Could you check a few things on this model? Use its own coordinates, in mm. A direction names the side the tool comes from. Round coordinates to 2 decimals unless told otherwise and drop trailing zeros. Order: outer loops, then holes, each group sorted by start corner. A loop starts at its lowest first (then second) coordinate and runs counter-clockwise, first axis right, second up. Notation, with made-up numbers: (-34.5, 81.25) - (-6.5, 81.25) arc R23 ccw to (-6.5, 100.25) - close; hole circle Ø10 at (-6.5, 35.5). An arc over 180 degrees is marked (long way). Return JSON: item names as keys, results as strings. Group by question number.
from build123d import *

# Parameters (mm, degrees)
SKETCH1_W                 = 100
SKETCH1_H                 = 126.094412
BOSS_EXTRUDE1_DEPTH       = 5
SLOTS_DEPTH               = 11
CUT_EXTRUDE5_DEPTH        = 3
CHAMFER2_SIZE             = 0.2
M5X0_8_TAPPED_HOLE2_D     = 4.2
SKETCH10_R                = 4.15
CUT_EXTRUDE4_DEPTH        = 5
M5X0_8_TAPPED_HOLE1_D     = 4.2
M5X0_8_TAPPED_HOLE1_DEPTH = 20
M5X0_8_TAPPED_HOLE1_TIP   = 1.2618073
CUT_EXTRUDE2_DEPTH        = 11
CUT_EXTRUDE3_DEPTH        = 11
FILLET1_R                 = 4
CHAMFER1_SIZE             = 2


with BuildPart() as part:
    # Sketch1 → Boss-Extrude1 (new body, symmetric)
    with BuildSketch(Plane(origin=(0, 0, 0), x_dir=(1, 0, 0), z_dir=(0, 1, 0))):
        with Locations((10, -5.047206)):
            Rectangle(SKETCH1_W, SKETCH1_H)
    extrude(amount=BOSS_EXTRUDE1_DEPTH, both=True)

    # Sketch3 → Slots (cut, through all)
    with BuildSketch(Plane(origin=(0, 5, 0), x_dir=(1, 0, 0), z_dir=(0, 1, 0))):
        with BuildLine():
            Line((-8.05, 0), (-8.05, -34.641016151))
            ThreePointArc((-8.05, -34.641016151), (0, -42.691016151), (8.05, -34.641016151))
            Line((8.05, -34.641016151), (8.05, 0))
            ThreePointArc((8.05, 0), (0, 8.05), (-8.05, 0))
        make_face()
        with BuildLine():
            Line((-11.95, 0), (-11.95, 20))
            ThreePointArc((-11.95, 20), (-8.449926035, 28.449926035), (0, 31.95))
            ThreePointArc((0, 31.95), (15.975, 27.669511651), (27.669511651, 15.975))
            ThreePointArc((27.669511651, 15.975), (38.666016151, 13.0284955), (41.612520652, 24.025))
            ThreePointArc((41.612520652, 24.025), (24.025, 41.612520652), (0, 48.05))
            ThreePointArc((0, 48.05), (-19.834345212, 39.834345212), (-28.05, 20))
            Line((-28.05, 20), (-28.05, 0))
            ThreePointArc((-28.05, 0), (-20, -8.05), (-11.95, 0))
        make_face()
    extrude(amount=-SLOTS_DEPTH, mode=Mode.SUBTRACT)

    # Sketch11 → Cut-Extrude5 (cut)
    with BuildSketch(Plane(origin=(0, 5, 0), x_dir=(1, 0, 0), z_dir=(0, 1, 0))):
        with BuildLine():
            Line((-10.15, 0), (-10.15, -34.641016151))
            ThreePointArc((-10.15, -34.641016151), (0, -44.791016151), (10.15, -34.641016151))
            Line((10.15, -34.641016151), (10.15, 0))
            ThreePointArc((10.15, 0), (0, 10.15), (-10.15, 0))
        make_face()
    extrude(amount=-CUT_EXTRUDE5_DEPTH, mode=Mode.SUBTRACT)

    # Chamfer2
    chamfer2_edges = [part.edges().sort_by_distance(p)[0] for p in [
        (0, 5, -10.15),
        (-10.15, 5, 17.320508076),
        (0, 5, 44.791016151),
        (10.15, 5, 17.320508076),
    ]]
    chamfer(chamfer2_edges, length=CHAMFER2_SIZE)

    # M5x0.8 Tapped Hole2 (through all)
    with Locations(Plane(origin=(0, 5, 0), x_dir=(1, 0, 0), z_dir=(0, 1, 0))):
        with Locations((-20, -34.641016151)):
            Hole(M5X0_8_TAPPED_HOLE2_D / 2)

    # Sketch10 → Cut-Extrude4 (cut)
    with BuildSketch(Plane(origin=(0, 5, 0), x_dir=(1, 0, 0), z_dir=(0, 1, 0))):
        with Locations((-20, -34.641016151)):
            Circle(SKETCH10_R)
    extrude(amount=-CUT_EXTRUDE4_DEPTH, mode=Mode.SUBTRACT)

    # M5x0.8 Tapped Hole1
    with Locations(Plane.XY.offset(68.094412)):
        with Locations((-15, 0), (35, 0)):
            Hole(M5X0_8_TAPPED_HOLE1_D / 2, depth=M5X0_8_TAPPED_HOLE1_DEPTH)
            with Locations((0, 0, -(M5X0_8_TAPPED_HOLE1_DEPTH + M5X0_8_TAPPED_HOLE1_TIP / 2))):  # 118° drill point
                Cone(0, M5X0_8_TAPPED_HOLE1_D / 2, M5X0_8_TAPPED_HOLE1_TIP, mode=Mode.SUBTRACT)

    # Sketch4 → Cut-Extrude2 (cut, through all)
    with BuildSketch(Plane(origin=(0, 5, 0), x_dir=(1, 0, 0), z_dir=(0, 1, 0))):
        Polygon((-40, 43), (-40, 58), (-25, 58), align=None)
    extrude(amount=-CUT_EXTRUDE2_DEPTH, mode=Mode.SUBTRACT)

    # Sketch5 → Cut-Extrude3 (cut, through all)
    with BuildSketch(Plane(origin=(0, 5, 0), x_dir=(1, 0, 0), z_dir=(0, 1, 0))):
        Polygon((25, 58), (60, 58), (60, 23), align=None)
    extrude(amount=-CUT_EXTRUDE3_DEPTH, mode=Mode.SUBTRACT)

    # Fillet1
    fillet1_edges = [part.edges().sort_by_distance(p)[0] for p in [
        (-25, 0, -58),
        (-40, 0, -43),
        (60, 0, -23),
        (25, 0, -58),
    ]]
    fillet(fillet1_edges, radius=FILLET1_R)

    # Chamfer1
    chamfer1_edges = [part.edges().sort_by_distance(p)[0] for p in [
        (60, 5, 23.375633125),
        (42.5, 5, -40.5),
        (0, 5, -58),
        (-32.5, 5, -50.5),
        (-40, 5, 13.375633125),
        (-39.69551813, 5, -42.87387948),
        (-24.87387948, 5, -57.69551813),
        (24.87387948, 5, -57.69551813),
        (59.69551813, 5, -22.87387948),
        (42.5, -5, -40.5),
        (-40, -5, 13.375633125),
        (-32.5, -5, -50.5),
        (0, -5, -58),
        (-39.69551813, -5, -42.87387948),
        (-24.87387948, -5, -57.69551813),
        (24.87387948, -5, -57.69551813),
        (59.69551813, -5, -22.87387948),
        (60, -5, 23.375633125),
    ]]
    chamfer(chamfer1_edges, length=CHAMFER1_SIZE)


solid = part.part
1) If I drill on line 1 along X through (y, z) = (0, 60.75); line 2 along Y through (x, z) = (35, 52.5); line 3 along Z through (x, y) = (-20, -3.05), over which ranges is the centre line in solid material (lowest first)? Write a range as from..to.
2) I want a section at B-B, the plane z = 5.5. List the corners of the cut face in (x, y) for me, plus the area to 3 significant figures.
3) I want a section at D-D, the plane x = 48. List the corners of the cut face in (y, z) for me, plus the area to 3 significant figures.
4) I want a section at C-C, the plane x = -20. List the corners of the cut face in (y, z) for me, plus the area to 3 significant figures.
5) Will these pins go through, and if not, where does the flat tip stop? pin 1 (0.8 mm diameter, centred on y = 4, z = 14, fed in from -X); pin 2 (7.5 mm diameter, centred on x = -20, z = 34.64, fed in from +Y); pin 3 (16 mm diameter, centred on x = -1.5, z = 5.5, fed in from +Y); pin 4 (6.5 mm diameter, centred on x = -18, z = 34.5, fed in from +Y).
6) For faces 4 (the cylindrical face through (-23.29, 2.54, 37.17)), 5 (the flat face through (-28.05, 0, -10)), 6 (the flat face through (60, 0, 24)), which set-ups out of +Z, -Z, +X, -X, +Y, -Y let a thin tool reach every point of the face, with its end or its side?
7) I want a section at A-A, the plane z = 57. List the corners of the cut face in (x, y) for me.
8) We'd pull the mould along X, two halves only. Please class faces 1 (the cylindrical face through (0.223, 3.42, -10.148)), 2 (the flat face through (-32, 0, -51)), 3 (the cylindrical face through (59.69, -0.04, -22.89)): +X half, -X half, draft (parallel to the pull), parting line (faces both ways), or undercut.
Outcome:
{
 "1": {"line 1": "-40..-17.1, -12.9..32.9, 37.1..60", "line 2": "-5..-2.1, 2.1..5", "line 3": "-57.95..-39.67, 8.05..32.54, 36.74..68.09"},
 "2": {"outline": "(-40, -3) - (-38, -5) - (-25.88, -5) - (-25.88, 5) - (-38, 5) - (-40, 3) - close; (-14.12, -5) - (-8.05, -5) - (-8.05, 2) - (-10.15, 2) - (-10.15, 4.8) - (-10.35, 5) - (-14.12, 5) - close; (8.05, -5) - (58, -5) - (60, -3) - (60, 3) - (58, 5) - (10.35, 5) - (10.15, 4.8) - (10.15, 2) - (8.05, 2) - close", "area": "701 mm^2"},
 "3": {"outline": "(-5, -32.17) - (-3, -35) - (3, -35) - (5, -32.17) - (5, 68.09) - (-5, 68.09) - close", "area": "1,030 mm^2"},
 "4": {"outline": "(-5, -56) - (-3, -58) - (3, -58) - (5, -56) - (5, -39.67) - (-5, -39.67) - close; (-5, 8.05) - (5, 8.05) - (5, 30.49) - (0, 30.49) - (0, 32.54) - (-5, 32.54) - close; (-5, 36.74) - (0, 36.74) - (0, 38.79) - (5, 38.79) - (5, 68.09) - (-5, 68.09) - close", "area": "717 mm^2"},
 "5": {"pin 1": "x = -39.4", "pin 2": "y = 0", "pin 3": "y = 2", "pin 4": "y = 5"},
 "6": {"face 4": "+Y", "face 5": "+Y, -Y", "face 6": "+Z, -Z, +X, +Y, -Y"},
 "7": {"outline": "(-40, -3) - (-38, -5) - (58, -5) - (60, -3) - (60, 3) - (58, 5) - (-38, 5) - (-40, 3) - close; hole circle Ø4.2 at (-15, 0); hole circle Ø4.2 at (35, 0)"},
 "8": {"face 1": "undercut", "face 2": "-X half", "face 3": "+X half"}
}
